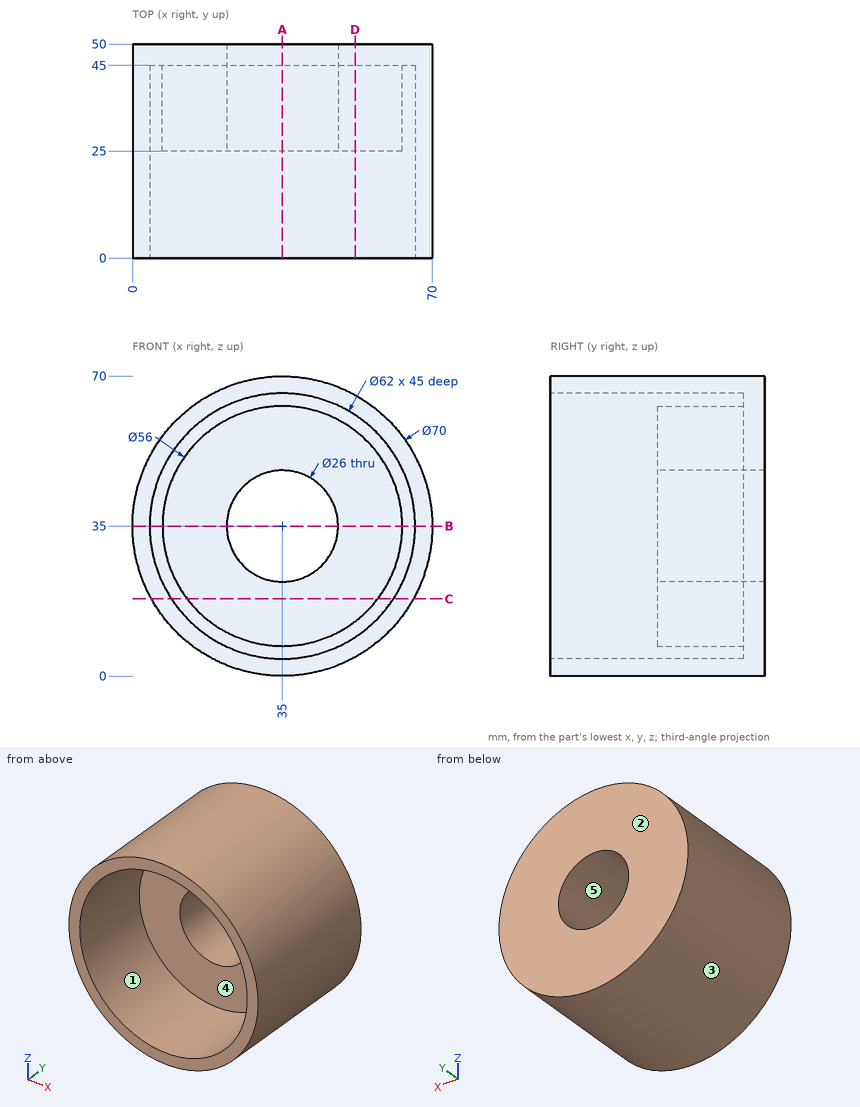
Source: three-view drawing plus pictorial views. Frame: mm from the lowest corner of the part. A direction names the side the tool comes from. Round coordinates to 2 decimals unless told otherwise and drop trailing zeros. Loops run counter-clockwise (first coordinate to the right, second up) from the corner with the lowest first, then second, coordinate; pieces in that order, holes last.
1. Section query C-C on z = 18. Output: boundary loops of the cut face in (x, y), and give its area (3 significant figures).
2. Contact query for flat-ended pins moving along their axis: pin 1 (6 mm diameter, centred on y = 25, z = 43, fed in from -X); pin 2 (6 mm diameter, centred on x = 27.5, y = 14.5, fed in from +Z); pin 3 (3 mm diameter, centred on y = 34.5, z = 24, fed in from +X); pin 4 (15.5 mm diameter, centred on x = 35, z = 35, fed in from +Y). Output: stop coordinate, or through.
3. Access query for the marked faces 4 and 5. Directions: +Z, -Z, +X, -X, +Y, -Y. A direction counts if a zero-diameter tool reaches every point of the face in a straight line with its end or side. Return the directions, or none.
4. Section query B-B on z = 35. Output: boundary loops of the cut face in (x, y), and give its area (3 significant figures).
5. Ray query, L1, parallel to Z at x = 35, y = 35.5; L2, parallel to Z at x = 35, y = 18.5. Return the intervals inside material, ascending.
6. Section query A-A on x = 35. Output: boundary loops of the cut face in (y, z), and give its area (3 significant figures).
7. Section query D-D on x = 52. Output: boundary loops of the cut face in (y, z), and give its area (3 significant figures).
8. Mould query, pull axis Z, two halves, no side actions, for the marked faces 1, 2 and 3. Classes: released by +Z, released by -Z, zero draft, split by the parting line, or undercut.
Answers below:
1. outline: (4.41, 0) - (9.08, 0) - (9.08, 45) - (12.75, 45) - (12.75, 25) - (57.25, 25) - (57.25, 45) - (60.92, 45) - (60.92, 0) - (65.59, 0) - (65.59, 50) - (4.41, 50) - close
1. area: 1,620 mm2
2. pin 1: stops at x = 0.36
2. pin 2: stops at z = 69.71
2. pin 3: stops at x = 68.69
2. pin 4: passes through
3. face 4: -Y
3. face 5: +Y, -Y
4. outline: (0, 0) - (4, 0) - (4, 45) - (7, 45) - (7, 25) - (22, 25) - (22, 50) - (0, 50) - close; (48, 25) - (63, 25) - (63, 45) - (66, 45) - (66, 0) - (70, 0) - (70, 50) - (48, 50) - close
4. area: 1,180 mm2
5. L1: z = 0 to 4, 7 to 22, 48 to 63, 66 to 70
5. L2: z = 0 to 4, 66 to 70
6. outline: (0, 0) - (50, 0) - (50, 22) - (25, 22) - (25, 7) - (45, 7) - (45, 4) - (0, 4) - close; (0, 66) - (45, 66) - (45, 63) - (25, 63) - (25, 48) - (50, 48) - (50, 70) - (0, 70) - close
6. area: 1,180 mm2
7. outline: (0, 4.41) - (50, 4.41) - (50, 65.59) - (0, 65.59) - (0, 60.92) - (45, 60.92) - (45, 57.25) - (25, 57.25) - (25, 12.75) - (45, 12.75) - (45, 9.08) - (0, 9.08) - close
7. area: 1,620 mm2
8. face 1: undercut
8. face 2: zero draft
8. face 3: split by the parting line
